from build123d import *

# Parameters (mm, degrees)
BOSS_EXTRUDE1_DEPTH      = 5.08
BOSS_EXTRUDE1_DEPTH_BACK = 0.278409343
SKETCH1_R                = 1.8415
CUT_EXTRUDE1_DEPTH       = 72.358313291
CUT_EXTRUDE1_DEPTH_BACK  = 72.358313291
BOSS_EXTRUDE2_DEPTH      = 0.635
FILLET2_R                = 12.7
CUT_EXTRUDE2_DEPTH       = 72.358313411
CUT_EXTRUDE2_DEPTH_BACK  = 72.358313411
FILLET3_R                = 25.4


with BuildPart() as part:
    # Sketch1 → Boss-Extrude1 (new, two sides: drawn at the far end of the back side and taken through both)
    with BuildSketch(Plane.XY.offset(-BOSS_EXTRUDE1_DEPTH_BACK)):
        with BuildLine():
            Line((-1.208443772, 47.324573258), (-1.208443772, 10.242675014))
            Line((-1.208443772, 10.242675014), (-4.452925719, 1.68904079))
            ThreePointArc((-4.452925719, 1.68904079), (-1.68904079, -4.452925719), (4.452925719, -1.68904079))
            Line((4.452925719, -1.68904079), (16.51, 18.415))
            ThreePointArc((16.51, 18.415), (13.107045256, 31.115), (16.51, 43.815))
            Line((16.51, 43.815), (16.51, 69.215))
            Line((16.51, 69.215), (11.43, 69.215))
            Line((11.43, 69.215), (-1.208443772, 47.324573258))
        make_face()
        Circle(SKETCH1_R, mode=Mode.SUBTRACT)
        with Locations((6.985, 18.415)):
            Circle(SKETCH1_R, mode=Mode.SUBTRACT)
    extrude(amount=BOSS_EXTRUDE1_DEPTH + BOSS_EXTRUDE1_DEPTH_BACK)

    # Sketch2 → Cut-Extrude1 (cut, two sides: drawn at the far end of the back side and taken through both)
    with BuildSketch(Plane(origin=(0, 0, -0.278409343), x_dir=(-1, 0, 0), z_dir=(0, 0, -1)).offset(-CUT_EXTRUDE1_DEPTH_BACK)):
        Polygon((-16.51, 64.442139164), (-15.24, 65.712139164), (-16.51, 66.982139164), align=None)
        Polygon((-16.51, 61.902139164), (-16.51, 59.362139164), (-15.24, 60.632139164), align=None)
        Polygon((-15.24, 55.415909985), (-16.51, 56.685909985), (-16.51, 54.145909985), align=None)
        Polygon((-16.51, 49.202139164), (-15.24, 50.472139164), (-16.51, 51.742139164), align=None)
        Polygon((-16.51, 43.849680806), (-15.24, 45.119680806), (-16.51, 46.389680806), align=None)
    extrude(amount=CUT_EXTRUDE1_DEPTH + CUT_EXTRUDE1_DEPTH_BACK, mode=Mode.SUBTRACT)

    # Sketch5 → Boss-Extrude2 (add)
    # profile 1 of 5: a face of its own
    with BuildSketch(Plane(origin=(0, 0, -0.278409343), x_dir=(-1, 0, 0), z_dir=(0, 0, -1))):
        Polygon((-11.43, 49.268745692), (-11.43, 50.883373857), (-9.418496835, 52.375422908), (-9.795276899, 52.676846958), (-11.43, 52.676846958), (-11.43, 53.962922908), (-6.35, 53.962922908), (-6.35, 52.676846958), (-8.660917722, 52.676846958), (-6.35, 50.897440313), (-6.35, 49.397353287), (-8.701107595, 51.338524173), align=None)
    # profile 2 of 5: a face of its own
    with BuildSketch(Plane(origin=(0, 0, -0.278409343), x_dir=(-1, 0, 0), z_dir=(0, 0, -1))):
        Polygon((-11.43, 43.931530503), (-11.43, 45.303009933), (-10.401139241, 45.658690313), (-10.401139241, 47.54560487), (-11.43, 47.901285249), (-11.43, 49.204441895), (-6.35, 47.323555819), (-6.35, 45.812416579), align=None)
        Polygon((-9.500886076, 45.963128604), (-7.647128165, 46.602147591), (-9.500886076, 47.241166579), align=None, mode=Mode.SUBTRACT)
    # profile 3 of 5: a face of its own
    with BuildSketch(Plane(origin=(0, 0, -0.278409343), x_dir=(-1, 0, 0), z_dir=(0, 0, -1))):
        with BuildLine():
            add(Edge.make_bspline(
                [(-7.945537975, 39.044441895), (-8.001893228, 39.045595729), (-8.114416057, 39.047899554), (-8.28200483, 39.072775037), (-8.447950006, 39.109194211), (-8.609957002, 39.161582728), (-8.764806034, 39.226372615), (-8.907675176, 39.307175215), (-9.039325299, 39.398356472), (-9.116222705, 39.470801449), (-9.154248418, 39.506625439)],
                knots=[0, 0, 0, 0, 1.018976149, 2.03455883, 3.059303171, 4.090371279, 5.111291766, 6.090739543, 7.055872052, 8, 8, 8, 8], degree=3))
            add(Edge.make_bspline(
                [(-9.154248418, 39.506625439), (-9.201805939, 39.55801623), (-9.296070219, 39.659878477), (-9.418570971, 39.826256442), (-9.522735706, 40.00129059), (-9.610286921, 40.186696086), (-9.676976835, 40.389424255), (-9.724895215, 40.612612286), (-9.752324851, 40.858668471), (-9.756124843, 41.030087139), (-9.758101266, 41.11924411)],
                knots=[0, 0, 0, 0, 0.948117162, 1.879273337, 2.792894651, 3.704383692, 4.651446974, 5.677657949, 6.792121143, 8, 8, 8, 8], degree=3))
            Line((-9.758101266, 41.11924411), (-9.758101266, 41.938112781))
            Line((-9.758101266, 41.938112781), (-11.43, 41.938112781))
            Line((-11.43, 41.938112781), (-11.43, 43.22418873))
            Line((-11.43, 43.22418873), (-6.35, 43.22418873))
            Line((-6.35, 43.22418873), (-6.35, 41.075035249))
            add(Edge.make_bspline(
                [(-6.35, 41.075035249), (-6.350776756, 40.997637205), (-6.35226824, 40.849021858), (-6.368729674, 40.63535844), (-6.394065089, 40.440645282), (-6.429937183, 40.263077028), (-6.478568776, 40.100769403), (-6.533724195, 39.948050161), (-6.602528473, 39.805953028), (-6.656105267, 39.717237318), (-6.682571203, 39.673413414)],
                knots=[0, 0, 0, 0, 1.27106079, 2.440619017, 3.517381815, 4.494852357, 5.412224011, 6.298180721, 7.159333057, 8, 8, 8, 8], degree=3))
            add(Edge.make_bspline(
                [(-6.682571203, 39.673413414), (-6.716741123, 39.624441403), (-6.784307056, 39.527606537), (-6.908159272, 39.40226874), (-7.043131438, 39.291772761), (-7.194439682, 39.202199788), (-7.360207545, 39.131182806), (-7.541414973, 39.079940069), (-7.738556134, 39.049817137), (-7.875098439, 39.046271184), (-7.945537975, 39.044441895)],
                knots=[0, 0, 0, 0, 0.969589194, 1.917218374, 2.854679868, 3.800052037, 4.766330684, 5.780154268, 6.854824506, 8, 8, 8, 8], degree=3))
        make_face()
        with BuildLine():
            add(Edge.make_bspline(
                [(-7.980704114, 40.394821642), (-7.94708576, 40.396040367), (-7.881091423, 40.398432779), (-7.786293373, 40.42106559), (-7.698560794, 40.457900068), (-7.620028501, 40.509101182), (-7.551714372, 40.570364624), (-7.492559182, 40.636019652), (-7.443946978, 40.706545052), (-7.421922651, 40.758113612), (-7.411012658, 40.783658667)],
                knots=[0, 0, 0, 0, 1.099448196, 2.158266167, 3.170681306, 4.20198982, 5.212085426, 6.167530276, 7.092265935, 8, 8, 8, 8], degree=3))
            add(Edge.make_bspline(
                [(-7.411012658, 40.783658667), (-7.398681248, 40.817631613), (-7.374423802, 40.884460703), (-7.349009707, 40.986535287), (-7.329727426, 41.086742841), (-7.322884819, 41.189157588), (-7.319312234, 41.298731496), (-7.315930195, 41.421655598), (-7.315672903, 41.560999172), (-7.314943057, 41.659128638), (-7.314556962, 41.711039996)],
                knots=[0, 0, 0, 0, 0.923484003, 1.816610051, 2.686736138, 3.528764097, 4.437155579, 5.490796045, 6.672608819, 8, 8, 8, 8], degree=3))
            Line((-7.314556962, 41.711039996), (-7.314556962, 41.938112781))
            Line((-7.314556962, 41.938112781), (-8.793544304, 41.938112781))
            Line((-8.793544304, 41.938112781), (-8.793544304, 41.559323224))
            add(Edge.make_bspline(
                [(-8.793544304, 41.559323224), (-8.793416885, 41.505386209), (-8.793174545, 41.402802255), (-8.784393416, 41.256060304), (-8.773143564, 41.124216394), (-8.756507529, 41.005510708), (-8.732152805, 40.898637133), (-8.695984985, 40.802354267), (-8.652914661, 40.713226884), (-8.613902833, 40.661532903), (-8.59460443, 40.635960882)],
                knots=[0, 0, 0, 0, 1.344391089, 2.556925957, 3.663619572, 4.642520217, 5.543736864, 6.38907055, 7.203104098, 8, 8, 8, 8], degree=3))
            add(Edge.make_bspline(
                [(-8.59460443, 40.635960882), (-8.57631846, 40.615730536), (-8.540475406, 40.576076235), (-8.478983071, 40.52504715), (-8.412749808, 40.483066813), (-8.340873581, 40.448470473), (-8.261518495, 40.425677511), (-8.175411224, 40.406665169), (-8.080697555, 40.397552624), (-8.014877557, 40.395754974), (-7.980704114, 40.394821642)],
                knots=[0, 0, 0, 0, 0.95676139, 1.87538582, 2.79551496, 3.705743042, 4.665608113, 5.687530201, 6.799376242, 8, 8, 8, 8], degree=3))
        make_face(mode=Mode.SUBTRACT)
    # profile 4 of 5: a face of its own
    with BuildSketch(Plane(origin=(0, 0, -0.278409343), x_dir=(-1, 0, 0), z_dir=(0, 0, -1))):
        Polygon((-7.314556962, 34.157353287), (-7.314556962, 35.764948224), (-11.43, 35.764948224), (-11.43, 37.051024173), (-7.314556962, 37.051024173), (-7.314556962, 38.65861911), (-6.35, 38.65861911), (-6.35, 34.157353287), align=None)
    # profile 5 of 5: a face of its own
    with BuildSketch(Plane(origin=(0, 0, -0.278409343), x_dir=(-1, 0, 0), z_dir=(0, 0, -1))):
        Polygon((-11.43, 28.691530503), (-11.43, 30.063009933), (-10.401139241, 30.418690313), (-10.401139241, 32.30560487), (-11.43, 32.661285249), (-11.43, 33.964441895), (-6.35, 32.083555819), (-6.35, 30.572416579), align=None)
        Polygon((-9.500886076, 30.723128604), (-7.647128165, 31.362147591), (-9.500886076, 32.001166579), align=None, mode=Mode.SUBTRACT)
    extrude(amount=BOSS_EXTRUDE2_DEPTH)

    # Fillet2
    fillet2_edges = [part.edges().sort_by_distance(p)[0] for p in [
        (16.51, 18.415, 2.400795328),
        (-1.208443772, 10.242675014, 2.400795328),
    ]]
    fillet(fillet2_edges, radius=FILLET2_R)

    # Sketch6 → Cut-Extrude2 (cut, two sides: drawn at the far end of the back side and taken through both)
    with BuildSketch(Plane(origin=(0, 0, -0.278409343), x_dir=(-1, 0, 0), z_dir=(0, 0, -1)).offset(-CUT_EXTRUDE2_DEPTH_BACK)):
        Polygon((-3.302, 55.136891036), (1.856635391, 55.136891036), (1.856635391, 24.765), (12.813790146, 19.47273461), (4.452925719, 1.68904079), (-2.532074281, 20.10404079), (-3.302, 22.133844959), align=None)
    extrude(amount=CUT_EXTRUDE2_DEPTH + CUT_EXTRUDE2_DEPTH_BACK, mode=Mode.SUBTRACT)

    # Fillet3
    fillet3_edges = [part.edges().sort_by_distance(p)[0] for p in [
        (3.302, 22.133844959, 2.400795328),
    ]]
    fillet(fillet3_edges, radius=FILLET3_R)


solid = part.part
Design review of the part built by this model. Coordinates are the model's own, in mm. A direction names the side the tool comes from. Round coordinates to 2 decimals unless told otherwise and drop trailing zeros. Write each loop counter-clockwise with the first axis right and the second up, starting at its lowest first coordinate (ties: lowest second). Pieces come first, ordered by that corner, then holes. Notation, with made-up numbers: (79, 31.5) - (88, 31.5) arc R23 cw to (88, 39.5) - close; hole circle Ø5 at (12.25, 32). An arc over 180 degrees is marked (long way). Use a Markdown table: item, result. Add a question column.
1. We need section D-D (y = 13.5). State the section outline as (x, z) points, then the cut area to 3 significant figures.
2. We need section B-B (x = 0). State the section outline as (y, z) points, then the cut area to 3 significant figures.
3. Clearance check with flat-ended pins moving along their axes: pin 1 (3 mm diameter, centred on y = 45, z = 2, fed in from -X); pin 2 (0.7 mm diameter, centred on y = 50.5, z = -0.5, fed in from +X); pin 3 (4 mm diameter, centred on x = 0, y = 0, fed in from +Z); pin 4 (0.7 mm diameter, centred on x = 7, z = -0.5, fed in from -Y). State where each tip first meets the part, or that it passes through.
4. For faces 1 (the face through (8.8, 46.6, -0.278)), 2 (the face through (14, 69.215, 2)), 3 (the face through (8.854, 29.645, -0.591)), 4 (the face through (15.88, 49.83, 2.44)), 5 (the face through (9, 52, -0.913)), list the 3-axis set-ups (+Z, -Z, +X, -X, +Y, -Y) from which the entire face can be reached by the end or side of a thin tool; tool diameter is ignored.
5. We need section C-C (z = 2.5). Count the separate pieces of the cut face and the enclosed holes in it, then the cut area to 3 significant figures.
6. Wall thickness on probe 1 along Z at (x, y) = (9.5, 58.5); probe 2 along Y at (x, z) = (7.5, 0.2); probe 3 along X at (y, z) = (18, 2.45): over which ranges is each line inside the solid? List them lowest first.
7. Mouldability with a two-part tool opening along X and no side actions: class faces 6 (the face through (8, 36, -0.913)), 7 (the face through (6.75, 20.24, 2.36)), 8 (the face through (16.51, 63, 2)) as +X half, -X half, draft (parallel to the pull), parting line (faces both ways), or undercut.
8. We need section A-A (y = 0). State the section outline as (x, z) points, then the cut area to 3 significant figures.
Output:
| question | item | result |
|---|---|---|
| 1 | outline | (0.03, -0.28) - (13.53, -0.28) - (13.53, 5.08) - (0.03, 5.08) - close |
| 1 | area | 72.4 mm2 |
| 2 | outline | (-4.76, -0.28) - (-1.84, -0.28) - (-1.84, 5.08) - (-4.76, 5.08) - close; (1.84, -0.28) - (13.43, -0.28) - (13.43, 5.08) - (1.84, 5.08) - close |
| 2 | area | 77.7 mm2 |
| 3 | pin 1 | stops at x = 3.3 |
| 3 | pin 2 | stops at x = 15.54 |
| 3 | pin 3 | stops at z = 5.08 |
| 3 | pin 4 | stops at y = 2.11 |
| 4 | face 1 | -Z |
| 4 | face 2 | +Z, -Z, +X, -X, +Y |
| 4 | face 3 | -Z, -X, -Y |
| 4 | face 4 | +Z, -Z, +X |
| 4 | face 5 | -Z, +X, -X, +Y, -Y |
| 5 | separate pieces | 1 |
| 5 | enclosed holes | 2 |
| 5 | area | 792 mm2 |
| 6 | probe 1 | z = -0.28 to 5.08 |
| 6 | probe 2 | y = 3.39 to 16.65, 20.18 to 62.41 |
| 6 | probe 3 | x = 1.73 to 5.19, 8.78 to 14.89 |
| 7 | face 6 | draft |
| 7 | face 7 | undercut |
| 7 | face 8 | +X half |
| 8 | outline | (-4.76, -0.28) - (-1.84, -0.28) - (-1.84, 5.08) - (-4.76, 5.08) - close; (1.84, -0.28) - (5.47, -0.28) - (5.47, 5.08) - (1.84, 5.08) - close |
| 8 | area | 35.1 mm2 |
